Autodesk Inventor part; units mm, degrees
ref_plane "YZ Plane" through (0, 0, 0) normal (1, 0, 0) x (0, 1, 0)
ref_plane "XZ Plane" through (0, 0, 0) normal (0, 1, 0) x (-1, 0, 0)
ref_plane "XY Plane" through (0, 0, 0) normal (0, 0, 1) x (1, 0, 0)
sketch "Sketch1" plane through (0, 0, 0) normal (0, 0, 1) x (1, 0, 0)
  circle A0 centre (0, 0) radius 17.78
  dimension "d0" = 35.56
extrude "Extrusion1" add sketch "Sketch1" along normal blind 15.875
sketch "Sketch2" plane through (0, 0, 15.875) normal (0, 0, 1) x (1, 0, 0)
  circle A0 centre (0, 0) radius 9.398
  dimension "d4" = 18.796
extrude "Extrusion2" add sketch "Sketch2" along normal blind 3.175
sketch "Sketch3" plane through (0, 0, 19.05) normal (0, 0, 1) x (1, 0, 0)
  circle A0 centre (0, 0) radius 3.175
  dimension "d7" = 6.35
extrude "Extrusion3" cut sketch "Sketch3" against normal blind 25.4
sketch "Sketch4" plane through (0, 0, 0) normal (0, 1, 0) x (-1, 0, 0)
  circle A0 centre (0, 7.9375) radius 2.0193
  line L0 (-17.78, 0) -> (17.78, 0)
  point P0 (0, 0)
  dimension "d10" = 4.0386
  dimension "d13" = 7.9375
extrude "Extrusion4" cut sketch "Sketch4" along normal blind 25.4
properties part number "Flywheel"
Build history of the part. All positions in model axes, mm. Give positions to 0.01 mm unless a question says otherwise; leave off trailing zeros. Loops run counter-clockwise (first coordinate to the right, second up) from the corner with the lowest first, then second, coordinate; pieces in that order, holes last. Notation, with made-up numbers: (78.25, 21) - (117.25, 21) arc R21 cw to (117.25, 46) - close; hole circle Ø6 at (40.25, -1.5). An arc over 180 degrees is marked (long way). Write item = value, one per line. Start each with the question number.
1) Pull direction Z, two halves, no side cores. Call faces 1 (the flat face through (8, -8, 15.875)), 2 (the cylindrical face through (0.44, 10.01, 9.91)), 3 (the flat face through (0, -4, 0)), 4 (the cylindrical face through (-1.22, -9.32, 17.44)): +Z half, -Z half, draft (parallel to the pull), parting line (faces both ways), or undercut.
2) Probe probe 1 along Z at (x, y) = (3, -12.5) (3 decimals); probe 2 along X at (y, z) = (-0.5, 4.25); probe 3 along X at (y, z) = (-1, 13.5). List the from-to ranges inside material, lowest first. Write a range as from..to.
3) Band-saw the part on C-C on z = 14.25. Give the cut face in (x, y) (3 decimals).
4) Band-saw the part on A-A on x = 0. Give the cut face in (y, z) (3 decimals).
5) Band-saw the part on B-B on y = 0. Give the cut face in (x, z) (3 decimals).
6) Drop flat-ended pins along their axis: pin 1 Ø5 at (x, y) = (8, -10) entering from +Z (3 decimals); pin 2 Ø2 at (y, z) = (-2, 13.5) entering from -X. Give the stop position or say it passes through.
Final values:
q1.face_1 = +Z half
q1.face_2 = undercut
q1.face_3 = -Z half
q1.face_4 = draft
q2.probe_1 = 0..15.875
q2.probe_2 = -17.77..-3.14, 3.14..17.77
q2.probe_3 = -17.75..-3.01, 3.01..17.75
q3.outline = circle Ø35.56 at (0, 0); hole circle Ø6.35 at (0, 0)
q4.outline = (-17.78, 0) - (-3.175, 0) - (-3.175, 19.05) - (-9.398, 19.05) - (-9.398, 15.875) - (-17.78, 15.875) - close; (3.175, 0) - (17.78, 0) - (17.78, 5.918) - (3.175, 5.918) - close; (3.175, 9.957) - (17.78, 9.957) - (17.78, 15.875) - (9.398, 15.875) - (9.398, 19.05) - (3.175, 19.05) - close
q5.outline = (-17.78, 0) - (-3.175, 0) - (-3.175, 19.05) - (-9.398, 19.05) - (-9.398, 15.875) - (-17.78, 15.875) - close; (3.175, 0) - (17.78, 0) - (17.78, 15.875) - (9.398, 15.875) - (9.398, 19.05) - (3.175, 19.05) - close
q6.pin_1 = 15.875
q6.pin_2 = -17.75
